Check sheet for the modelled part. Datum: model origin and axes. Units: mm. A direction names the side the tool comes from. Round coordinates to 2 decimals unless told otherwise and drop trailing zeros. Write each loop counter-clockwise with the first axis right and the second up, starting at its lowest first coordinate (ties: lowest second). Pieces come first, ordered by that corner, then holes.
Item 1: Go/stop test with flat-tipped pins: pin 1 Ø2.5 at (y, z) = (-2, 107) entering from +X; pin 2 Ø1.5 at (y, z) = (-1.5, 108) entering from -X; pin 3 Ø2 at (x, y) = (-1, -2) entering from +Z. Record where each tip stops, or that it passes through.
Item 2: Release check for a two-part mould opening along Z. For faces 6 (the flat face through (5.439, -2, 2)), 7 (the cylindrical face through (3.417, -1.452, 106.343)), 8 (the flat face through (-1, -1, 105)) record: +Z half, -Z half, draft (parallel to the pull), parting line (faces both ways), or undercut.
Item 3: Cross-section at B-B on x = 6.5. Enter the section's corners in (y, z), plus the area to 3 significant figures.
Item 4: Tool access check on faces 1 (the flat face through (0.439, -2, 107)), 2 (the flat face through (6, -1, 5)), 3 (the flat face through (3, 1.013, 54)), 4 (the flat face through (0.439, -2, 2)), 5 (the flat face through (6, -1, 105)). Record the directions out of +Z, -Z, +X, -X, +Y, -Y that give a thin tool (end or side, any length) a straight path to the whole face; none if there is none.
Item 5: Material ranges on line 1 (Z direction, x = 3, y = -0.9); line 2 (Z direction, x = 2.25, y = -1.8); line 3 (Z direction, x = 0, y = -2.7), recorded low to high.
Item 6: Cross-section at A-A on y = -1.75. Enter the section's corners in (x, z), plus the area to 3 significant figures.
from build123d import *

# Parameters (mm, degrees)
SKETCH1_W           = 5
SKETCH1_H           = 5
BOSS_EXTRUDE1_DEPTH = 110
SKETCH2_W           = 2
SKETCH2_H           = 100
BOSS_EXTRUDE2_DEPTH = 5
BOSS_EXTRUDE3_DEPTH = 5


with BuildPart() as part:
    # Sketch1 → Boss-Extrude1 (new body)
    with BuildSketch(Plane.XY):
        with Locations((2.938510718, -1.487078427)):
            Rectangle(SKETCH1_W, SKETCH1_H)
    extrude(amount=BOSS_EXTRUDE1_DEPTH)

    # Sketch2 → Boss-Extrude2 (add)
    with BuildSketch(Plane(origin=(0, 1.012921573, 0), x_dir=(1, 0, 0), z_dir=(0, 1, 0))):
        with Locations((6.438510718, -55)):
            Rectangle(SKETCH2_W, SKETCH2_H)
    extrude(amount=-BOSS_EXTRUDE2_DEPTH)

    # Sketch3 → Boss-Extrude3 (add)
    with BuildSketch(Plane(origin=(0, 1.012921573, 0), x_dir=(1, 0, 0), z_dir=(0, 1, 0))):
        Polygon((0.438510718, -5.009089169), (-1.561489282, -5), (-1.561489282, -105), (0.438510718, -105), align=None)
    extrude(amount=-BOSS_EXTRUDE3_DEPTH)

    # Sketch6 → M3 Tapped Hole1 (revolve, cut)
    with BuildSketch(Plane(origin=(2.938510718, 1.012921573, 2.502272292), x_dir=(0, 0, 1), z_dir=(1, 0, 0))):
        Polygon((0, 0), (0, 8.751075774), (1.25, 8), (1.25, 0), align=None)
    m3_tapped_hole1 = revolve(axis=Axis((2.938510718, 7.362921573, 2.502272292), (0, -1, 0)), mode=Mode.SUBTRACT)

    # Mirror1: M3 Tapped Hole1 across plane
    add(m3_tapped_hole1.mirror(Plane(origin=(0, 0, 55), x_dir=(1, 0, 0), z_dir=(0, 0, -1))), mode=Mode.SUBTRACT)


solid = part.part
Response values:
1. pin 1: stops at x = 5.44
1. pin 2: stops at x = 0.44
1. pin 3: stops at z = 105
2. face 6: draft
2. face 7: undercut
2. face 8: +Z half
3. outline: (-3.99, 5) - (1.01, 5) - (1.01, 105) - (-3.99, 105) - close
3. area: 500 mm2
4. face 1: +Z, -X, +Y, -Y
4. face 2: -Z, +X, +Y, -Y
4. face 3: +Z, -Z, +X, -X, +Y
4. face 4: -Z, -X, +Y, -Y
4. face 5: +Z, +X, +Y, -Y
5. line 1: z = 0 to 1.25, 3.75 to 106.25, 108.75 to 110
5. line 2: z = 0 to 1.46, 3.55 to 106.45, 108.54 to 110
5. line 3: z = 5.01 to 105
6. outline: (-1.56, 5) - (0.44, 5.01) - (0.44, 0) - (5.44, 0) - (5.44, 5) - (7.44, 5) - (7.44, 105) - (5.44, 105) - (5.44, 110) - (0.44, 110) - (0.44, 105) - (-1.56, 105) - close; hole circle Ø2.5 at (2.94, 2.5); hole circle Ø2.5 at (2.94, 107.5)
6. area: 940 mm2
